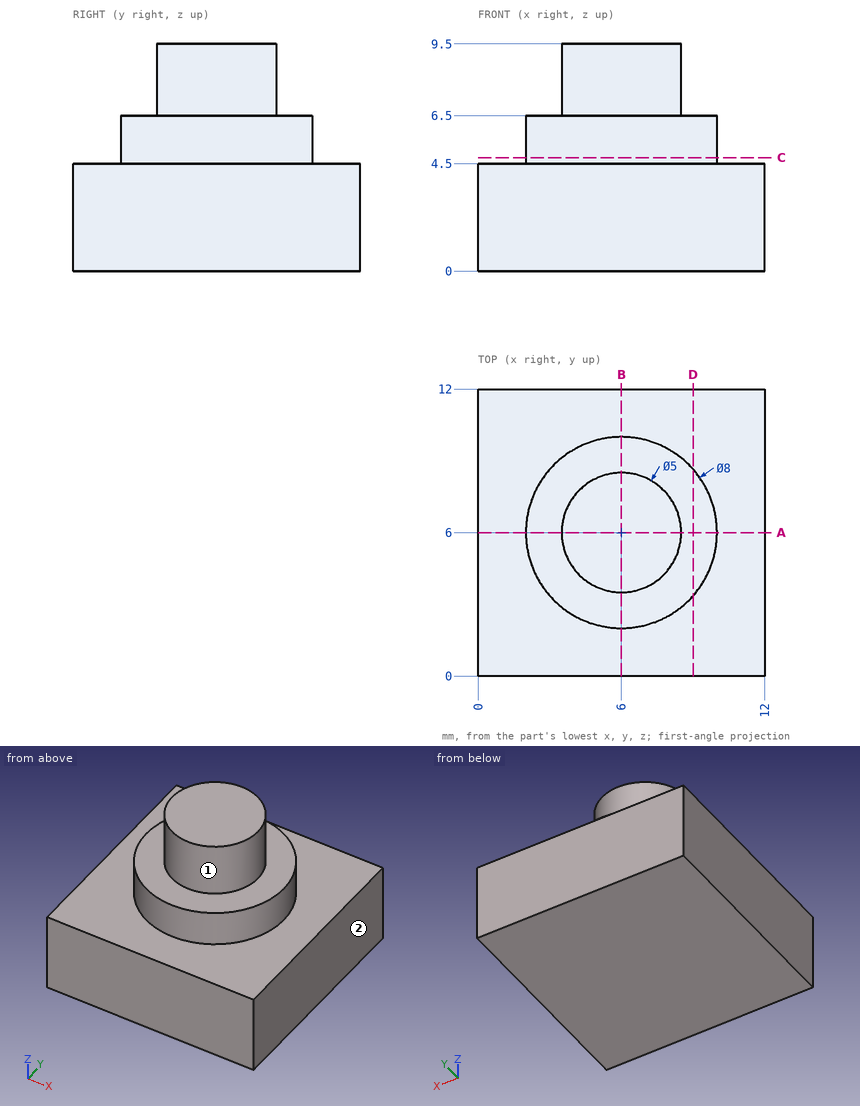
Can you work these out from the drawing? Everything is in mm from the part's minimum corner. A direction names the side the tool comes from. Round coordinates to 2 decimals unless told otherwise and drop trailing zeros. Loops run counter-clockwise (first coordinate to the right, second up) from the corner with the lowest first, then second, coordinate; pieces in that order, holes last. Notation, with made-up numbers: (49, 9) -> (69, 9) arc R30 cw to (69, 35) -> close; hole circle Ø6 at (30, -16). An arc over 180 degrees is marked (long way). Use CSV: the item, a comma, the result in double quotes.
(1) If I drill on probe 1 along Z at (x, y) = (1, 6.75); probe 2 along Z at (x, y) = (8, 3.75); probe 3 along Y at (x, z) = (6.25, 7), over which ranges is the centre line in solid material (lowest first)? Write a range as [from, to].
Return value:
probe 1,"z = [0, 4.5]"
probe 2,"z = [0, 6.5]"
probe 3,"y = [3.51, 8.49]"
(2) Suppose I cut it at A-A on y = 6. Write out the boundary of the cut face in (x, z), plus the area to 3 significant figures.
Return value:
outline,"(0, 0) -> (12, 0) -> (12, 4.5) -> (10, 4.5) -> (10, 6.5) -> (8.5, 6.5) -> (8.5, 9.5) -> (3.5, 9.5) -> (3.5, 6.5) -> (2, 6.5) -> (2, 4.5) -> (0, 4.5) -> close"
area,"85.0 mm²"
(3) Suppose I cut it at D-D on x = 9. Write out the boundary of the cut face in (y, z), plus the area to 3 significant figures.
Return value:
outline,"(0, 0) -> (12, 0) -> (12, 4.5) -> (8.65, 4.5) -> (8.65, 6.5) -> (3.35, 6.5) -> (3.35, 4.5) -> (0, 4.5) -> close"
area,"64.6 mm²"
(4) For the marked faces 1 and 2, which set-ups out of +Z, -Z, +X, -X, +Y, -Y let a thin tool reach every point of the face, with its end or its side?
Return value:
face 1,"+Z"
face 2,"+Z, -Z, +X, +Y, -Y"
(5) Will this pin go through, and if not, where does the flat tip stop? pin 1 Ø1 at (x, y) = (10, 9.5) entering from +Z.
Return value:
pin 1,"stops at z = 4.5"
(6) Suppose I cut it at C-C on z = 4.75. Write out the boundary of the cut face in (x, y), plus the area to 3 significant figures.
Return value:
outline,"circle Ø8 at (6, 6)"
area,"50.3 mm²"
